from build123d import *

# Parameters (mm, degrees)
F1_DEPTH = 10
F3_DEPTH = 6
F2_W     = 2
F2_H     = 2.5
F2_W_2   = 3
F4_DEPTH = 6
F6_W     = 3
F6_H     = 3


with BuildPart() as f1:
    # F0 (on Front) → F1 (new body)
    with BuildSketch(Plane.XZ):
        Polygon((-22.397178, 0), (-28.397178, 0), (-28.397178, -2), (-20.397178, -2), (-20.397178, 5), (13.602822, 5), (15.602822, 5), (15.602822, 0), (9.602822, 0), (9.602822, -2), (18.602822, -2), (18.602822, 7), (-22.397178, 7), align=None)
    extrude(amount=F1_DEPTH)

    # F2 (on face) → F3 (cut)
    with BuildSketch(Plane.XZ.offset(10)):
        Polygon((-20.397178, 0), (-22.397178, 0), (-28.397178, 0), (-28.397178, -2), (-20.397178, -2), align=None)
        Polygon((18.602822, -2), (18.602822, 0), (15.602822, 0), (9.602822, 0), (9.602822, -2), align=None)
    extrude(amount=-F3_DEPTH, mode=Mode.SUBTRACT)

    # F2 (on face) → F4 (cut)
    with BuildSketch(Plane.XZ.offset(10)):
        with Locations((-21.397178, 1.25)):
            Rectangle(F2_W, F2_H)
        with Locations((17.102822, 1.25)):
            Rectangle(F2_W_2, F2_H)
    extrude(amount=-F4_DEPTH, mode=Mode.SUBTRACT)

    # F7: sweep along a path in F5
    with BuildLine(Plane.YZ) as f7_path:
        Line((0, 7.219068), (-5, 7.219068))
        ThreePointArc((-5, 7.219068), (-8.535534, 8.683534), (-10, 12.219068))
        Line((-10, 12.219068), (-10, 17.219068))
        ThreePointArc((-10, 17.219068), (-8.535534, 20.754602), (-5, 22.219068))
        Line((-5, 22.219068), (0, 22.219068))
    # F6 (on Front) → F7 (sweep)
    with BuildSketch(Plane.XZ):
        with Locations((0, 7.219068)):
            Rectangle(F6_W, F6_H)
    sweep(path=f7_path.line)

    # F8: F1 across plane


with BuildPart() as f1_1:
    add(f1.part)
    add(f1.part.mirror(Plane.XZ))


solid = f1_1.part
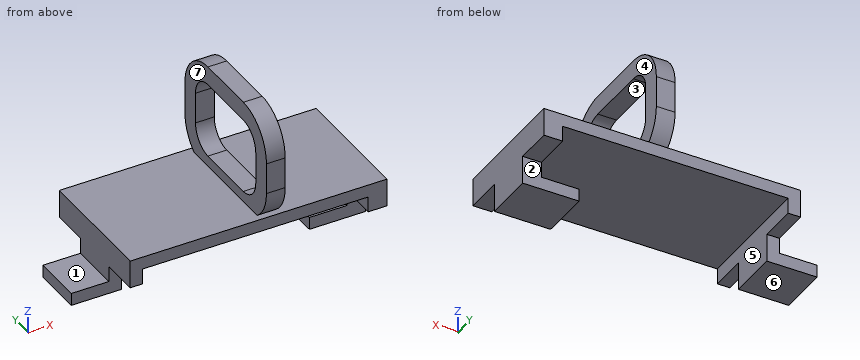
Geometry: final body of the model. Coordinates: model frame, mm. Face numbers are marked on the shaded views. A direction names the side the tool comes from. Give positions to 0.01 mm unless a question says otherwise; leave off trailing zeros. Write each loop counter-clockwise with the first axis right and the second up, starting at its lowest first coordinate (ties: lowest second). Pieces come first, ordered by that corner, then holes. Notation, with made-up numbers: (86.5, 9.5) -> (113.5, 9.5) arc R14 cw to (113.5, 32.5) -> close; hole circle Ø7 at (86, 2). An arc over 180 degrees is marked (long way). Answer as a JSON object with one key per item and string values.
1. Mould query, pull axis X, two halves, no side actions, for the marked faces 5, 6 and 7. Classes: pulls with the +X half, pulls with the -X half, needs draft (parallel to the pull), parting line crosses it, or undercut.
Ans:
{"face 5": "undercut", "face 6": "needs draft", "face 7": "pulls with the -X half"}
2. Cut plane C-C on z = 1. Output: boundary loops of the cut face in (x, y).
Ans:
{"outline": "(-22.4, -4) -> (-20.4, -4) -> (-20.4, 4) -> (-22.4, 4) -> close; (15.6, -4) -> (18.6, -4) -> (18.6, 4) -> (15.6, 4) -> close"}
3. Access query for the marked faces 1, 2, 3 and 4. Directions: +Z, -Z, +X, -X, +Y, -Y. A direction counts if a zero-diameter tool reaches every point of the face in a straight line with its end or side. Return the directions, or none.
Ans:
{"face 1": "+Z, -X, +Y, -Y", "face 2": "-Z, +X, -X, +Y", "face 3": "+X, -X", "face 4": "+Z, +X, +Y, -Y"}
4. Cut plane D-D on z = 19. Output: boundary loops of the cut face in (x, y), and give its area (3 significant figures).
Ans:
{"outline": "(-1.5, -11.25) -> (1.5, -11.25) -> (1.5, -8.01) -> (-1.5, -8.01) -> close; (-1.5, 8.01) -> (1.5, 8.01) -> (1.5, 11.25) -> (-1.5, 11.25) -> close", "area": "19.4 mm^2"}
5. Ray query, probe 1 along X at (y, z) = (2.25, 1.5); probe 2 along X at (y, z) = (-4.75, 5.75); probe 3 along Y at (x, z) = (-10.5, 5.75). Return the intervals inside material, ascending. Write a range as from..to.
Ans:
{"probe 1": "x = -22.4..-20.4, 15.6..18.6", "probe 2": "x = -22.4..18.6", "probe 3": "y = -10..10"}
6. Cut plane A-A on x = -0.5. Output: boundary loops of the cut face in (y, z), and give its area (3 significant figures).
Ans:
{"outline": "(-11.5, 12.22) arc R6.5 ccw to (-8.87, 7) -> (-10, 7) -> (-10, 5) -> (10, 5) -> (10, 7) -> (8.87, 7) arc R6.5 ccw to (11.5, 12.22) -> (11.5, 17.22) arc R6.5 ccw to (5, 23.72) -> (-5, 23.72) arc R6.5 ccw to (-11.5, 17.22) -> close; hole (-8.5, 12.22) arc R3.5 ccw to (-5, 8.72) -> (5, 8.72) arc R3.5 ccw to (8.5, 12.22) -> (8.5, 17.22) arc R3.5 ccw to (5, 20.72) -> (-5, 20.72) arc R3.5 ccw to (-8.5, 17.22) -> close", "area": "205 mm^2"}
7. Cut plane B-B on y = -0.5. Output: boundary loops of the cut face in (x, z), and give its area (3 significant figures).
Ans:
{"outline": "(-28.4, -2) -> (-20.4, -2) -> (-20.4, 5) -> (15.6, 5) -> (15.6, 0) -> (9.6, 0) -> (9.6, -2) -> (18.6, -2) -> (18.6, 7) -> (1.5, 7) -> (1.5, 8.72) -> (-1.5, 8.72) -> (-1.5, 7) -> (-22.4, 7) -> (-22.4, 0) -> (-28.4, 0) -> close; (-1.5, 20.72) -> (1.5, 20.72) -> (1.5, 23.72) -> (-1.5, 23.72) -> close", "area": "155 mm^2"}
8. Contact query for flat-ended pins moving along their axis: pin 1 (8 mm diameter, centred on x = -10, z = 6.5, fed in from -Y); pin 2 (1 mm diameter, centred on x = -6, y = -6.5, fed in from +Z); pin 3 (1.5 mm diameter, centred on x = -21.5, y = 8, fed in from -Z). Output: stop coordinate, or through.
Ans:
{"pin 1": "stops at y = -10", "pin 2": "stops at z = 7", "pin 3": "stops at z = 2.5"}
